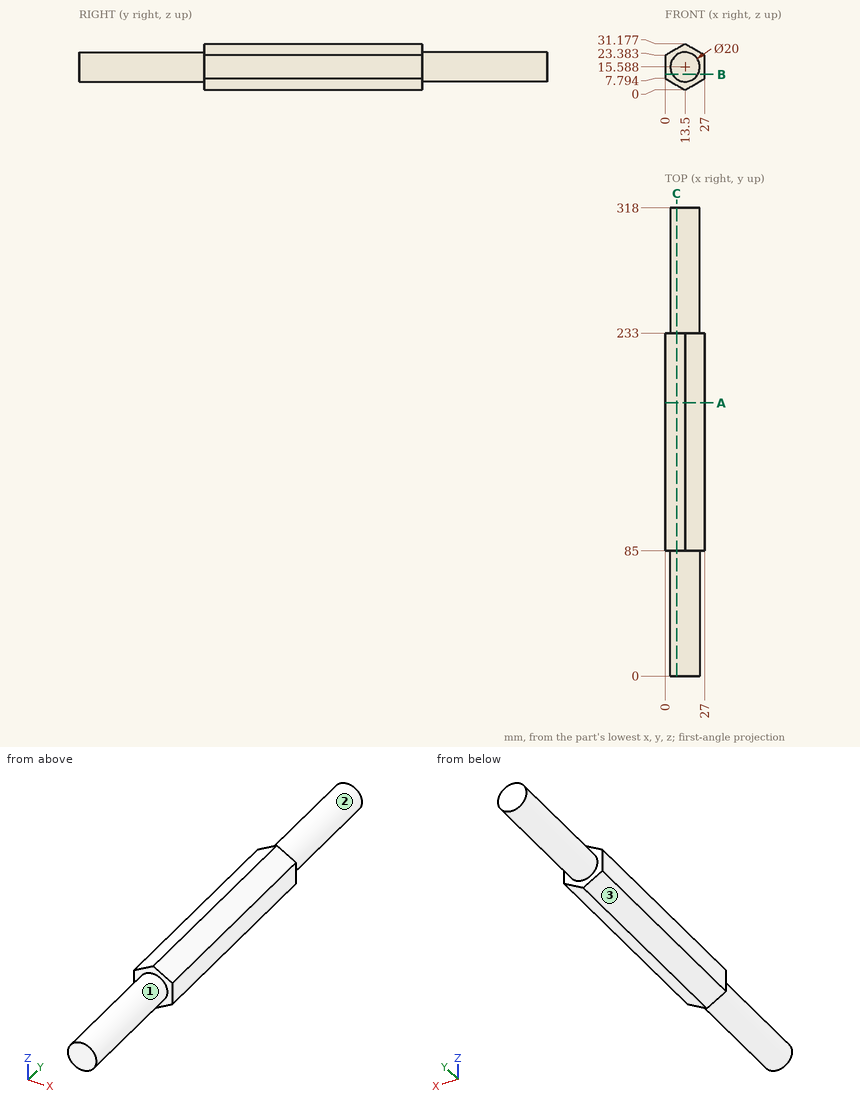
Verification items for this drawing (mm, ordinates from the low corner). A direction names the side the tool comes from. Coordinates: 2 decimals unless noted, no trailing zeros. Order: outer loops, then holes, each group sorted by start corner. A loop starts at its lowest first (then second) coordinate and runs counter-clockwise, first axis right, second up. Notation, with made-up numbers: M -17.5,71.25 L 23.5,71.25 A23 cw 23.5,107.25 Z; hole C 1,-37 d11. An arc over 180 degrees is marked long. Answer as a JSON object with one key per item and string values.
Q1. Cross-section at C-C on x = 7.75. Record the cut outline in (y, z).
Results are:
{"outline": "M 0,7.41 L 85,7.41 L 85,3.32 L 233,3.32 L 233,7.41 L 318,7.41 L 318,23.77 L 233,23.77 L 233,27.86 L 85,27.86 L 85,23.77 L 0,23.77 Z"}
Q2. Cross-section at B-B on z = 10.5. Record the cut outline in (x, y).
Results are:
{"outline": "M 0,85 L 4.89,85 L 4.89,0 L 22.11,0 L 22.11,85 L 27,85 L 27,233 L 22.11,233 L 22.11,318 L 4.89,318 L 4.89,233 L 0,233 Z"}
Q3. Cross-section at A-A on y = 185.5. Record the cut outline in (x, z) (1 decimal), and give its area (3 significant figures).
Results are:
{"outline": "M 0,7.8 L 13.5,0 L 27,7.8 L 27,23.4 L 13.5,31.2 L 0,23.4 Z", "area": "631 mm²"}
Q4. Scan lines: line 1 (Y direction, x = 23.25, z = 23.5); line 2 (Z direction, x = 14.5, y = 291); line 3 (X direction, y = 263.5, z = 15.5). Record each from-to range of solid material in increasing order.
Results are:
{"line 1": "y = 85 to 233", "line 2": "z = 5.64 to 25.54", "line 3": "x = 3.5 to 23.5"}
Q5. Depth check by flat-ended pin: pin 1 Ø4 at (x, y) = (7.5, 67.5) entering from +Z; pin 2 Ø8 at (y, z) = (45, 15) entering from +X; pin 3 Ø12 at (x, z) = (3.5, 27.5) entering from -Y; pin 4 Ø12 at (x, y) = (5.5, 111) entering from -Z (1 decimal). Enter the tip coordinate at first touch or a pass-through.
Results are:
{"pin 1": "stops at z = 24.75", "pin 2": "stops at x = 23.5", "pin 3": "stops at y = 0", "pin 4": "stops at z = 1.2"}
Q6. Tool access check on the marked faces 1, 2 and 3. Record the directions out of +Z, -Z, +X, -X, +Y, -Y that give a thin tool (end or side, any length) a straight path to the whole face; none if there is none.
Results are:
{"face 1": "-Y", "face 2": "+Y", "face 3": "-Z, -X, +Y, -Y"}
